Check sheet for the drawn part. Datum: minimum x, y, z corner. Units: mm. A direction names the side the tool comes from. Coordinates: 2 decimals unless noted, no trailing zeros. Order: outer loops, then holes, each group sorted by start corner. A loop starts at its lowest first (then second) coordinate and runs counter-clockwise, first axis right, second up. Notation, with made-up numbers: M 79.25,31 L 112.25,31 A16 ccw 112.25,62 Z; hole C 14.25,12 d8. An arc over 180 degrees is marked long. Use one line per item in the form item = value. Start each with the question number.
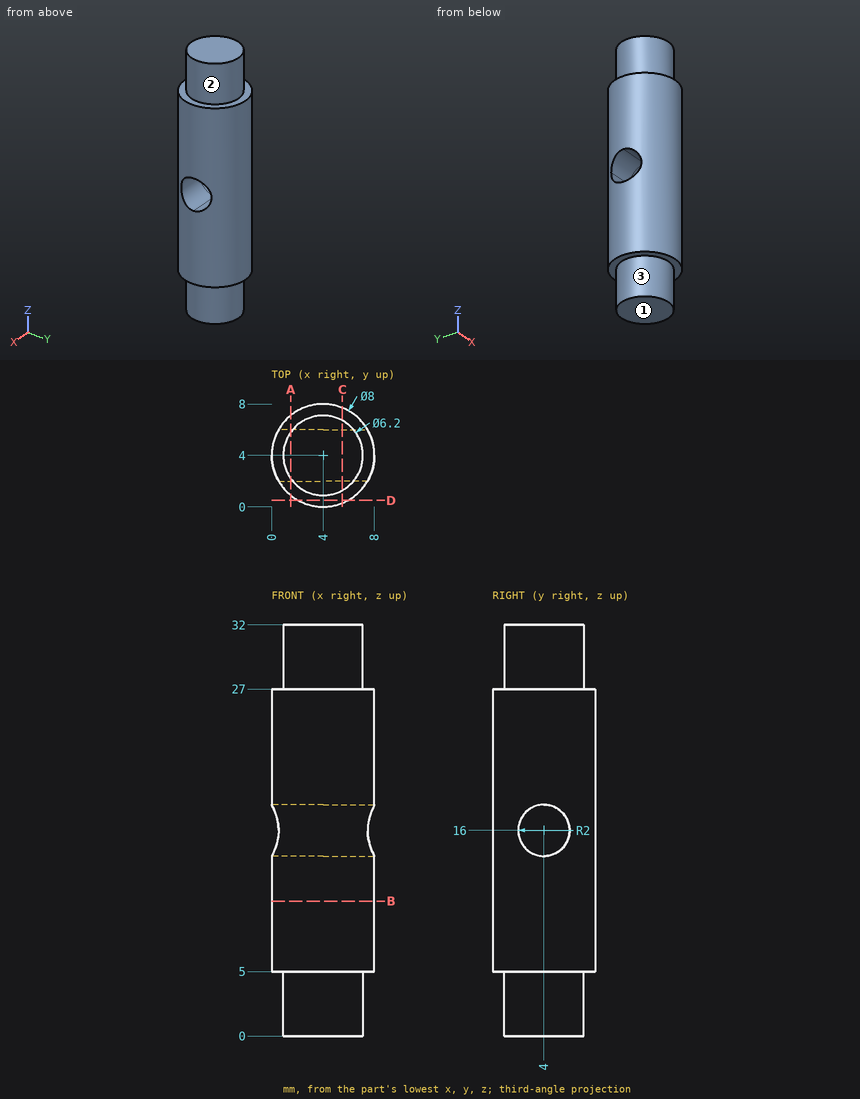
1. Depth check by flat-ended pin: P1, Ø3, axis at y = 6, z = 10, coming from the -X side; P2, Ø2, axis at y = 2.5, z = 3.5, coming from the +X side; P3, Ø1, axis at x = 5.5, z = 15, coming from the -Y side. Enter the tip coordinate at first touch or a pass-through.
2. Cross-section at A-A on x = 1.5. Enter the section's corners in (y, z).
3. Material ranges on line 1 along Z through (x, y) = (2.75, 3); line 2 along Z through (x, y) = (3, 2.25); line 3 along Z through (x, y) = (6.5, 1.75), recorded low to high.
4. Tool access check on the marked faces 1, 2 and 3. Record the directions out of +Z, -Z, +X, -X, +Y, -Y that give a thin tool (end or side, any length) a straight path to the whole face; none if there is none.
5. Cross-section at B-B on z = 10.5. Enter the section's corners in (x, y).
6. Cross-section at C-C on x = 5.5. Enter the section's corners in (y, z).
7. Cross-section at D-D on y = 0.5. Enter the section's corners in (x, z).
Final values:
q1.P1 = 0.03
q1.P2 = 7.06
q1.P3 = 0.13
q2.outline = M 0.88,5 L 2.17,5 L 2.17,0 L 5.83,0 L 5.83,5 L 7.12,5 L 7.12,27 L 5.83,27 L 5.83,32 L 2.17,32 L 2.17,27 L 0.88,27 Z; hole C 4,16 d4
q3.line_1 = 0 to 14.27, 17.73 to 32
q3.line_2 = 0 to 15.03, 16.97 to 32
q3.line_3 = 5 to 27
q4.face_1 = -Z, +X, -X, +Y, -Y
q4.face_2 = +Z
q4.face_3 = -Z
q5.outline = C 4,4 d8
q6.outline = M 0.29,5 L 1.29,5 L 1.29,0 L 6.71,0 L 6.71,5 L 7.71,5 L 7.71,27 L 6.71,27 L 6.71,32 L 1.29,32 L 1.29,27 L 0.29,27 Z; hole C 4,16 d4
q7.outline = M 2.06,5 L 5.94,5 L 5.94,27 L 2.06,27 Z
